Design review of the part built by this model. Coordinates are the model's own, in mm. A direction names the side the tool comes from. Coordinates: 2 decimals unless noted, no trailing zeros. Write each loop counter-clockwise with the first axis right and the second up, starting at its lowest first coordinate (ties: lowest second). Pieces come first, ordered by that corner, then holes.
Q1. The part is to be moulded in two halves that separate along X. For faces 3 (the face through (-1.5, -1.1, 1.5)), 4 (the face through (0, 2, 1)), 5 (the face through (-1.14, -1.07, 0.86)), say which applies: +X half, -X half, draft (parallel to the pull), parting line (faces both ways), or undercut.
Q2. Add section B-B, the plane z = 1.4. Give the boundary of the cut face in (x, y), plus the area to 3 significant figures.
Q3. Add section A-A, the plane z = 0.7. Give the boundary of the cut face in (x, y), plus the area to 3 significant figures.
Q4. To check wall thickness, follow probe 1 along Y at (x, z) = (-0.2, 0.15); probe 2 along Y at (x, z) = (-0.4, 0.6); probe 3 along X at (y, z) = (0.1, 1.05). State the ranges of each line that lie inside material, in increasing order.
Q5. Machinability: for faces 1 (the face through (-2.19, -2.05, 0.49)), 2 (the face through (2, 0, 1)), which of the approach directions +Z, -Z, +X, -X, +Y, -Y give a long, thin tool a straight path to every point of the face, cutting with its end or side? Answer none if there is none.
from build123d import *

# Parameters (mm, degrees)
F1_DEPTH = 1.5
F4_R     = 0.5


with BuildPart() as f1:
    # F0 (on Top) → F1 (new body)
    with BuildSketch(Plane.XY):
        with BuildLine():
            Line((0, 1.5), (0, 3))
            ThreePointArc((0, 3), (-2.12132, -2.12132), (3, 0))
            Line((3, 0), (1.5, 0))
            ThreePointArc((1.5, 0), (-1.06066, -1.06066), (0, 1.5))
        make_face()
    extrude(amount=F1_DEPTH)

    # F2 (on face) → F3 (revolve, cut)
    with BuildSketch(Plane.YZ):
        with BuildLine():
            ThreePointArc((1.558824, 0.264706), (1.514929, 0.378732), (1.5, 0.5))
            Line((1.5, 0.5), (1.5, 0))
            Line((1.5, 0), (1.7, 0))
            Line((1.7, 0), (1.558824, 0.264706))
        make_face()
        with BuildLine():
            Line((1.7, 1.5), (1.5, 1.5))
            Line((1.5, 1.5), (1.5, 0.5))
            ThreePointArc((1.5, 0.5), (1.502701, 0.551896), (1.510773, 0.603232))
            Line((1.510773, 0.603232), (1.7, 1.5))
        make_face()
    revolve(axis=Axis((0, 0, 0.75), (0, 0, 1)), mode=Mode.SUBTRACT)

    # F4
    f4_edges = [f1.edges().sort_by_distance(p)[0] for p in [
        (-2.12132, -2.12132, 1.5),
    ]]
    fillet(f4_edges, radius=F4_R)


solid = f1.part
Here are the results:
1. face 3: draft
1. face 4: +X half
1. face 5: undercut
2. outline: (0, 1.68) - (0, 2.8) arc R2.8 ccw (long way) to (2.8, 0) - (1.68, 0) arc R1.68 cw (long way) to start
2. area: 11.8 mm2
3. outline: (0, 1.53) - (0, 3) arc R3 ccw (long way) to (3, 0) - (1.53, 0) arc R1.53 cw (long way) to start
3. area: 15.7 mm2
4. probe 1: y = -2.99 to -1.61, 1.61 to 2.99
4. probe 2: y = -2.97 to -1.46, 1.46 to 2.97
4. probe 3: x = -3 to -1.6
5. face 1: +Z, -Z
5. face 2: +Z, -Z, +X, +Y
